Answer from the drawing. Dimensions are ordinates in mm from the lowest x, y and z of the part. A direction names the side the tool comes from. Coordinates: 2 decimals unless noted, no trailing zeros.
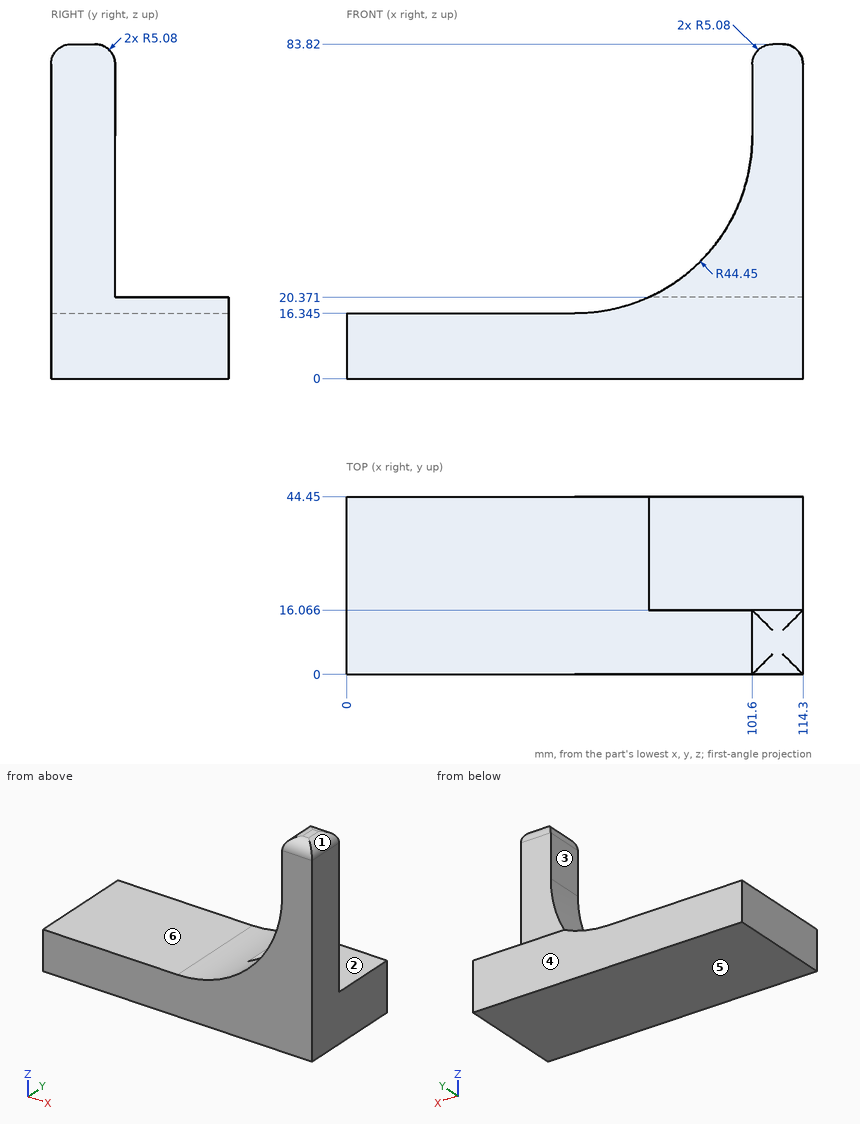
Item 1: Given pin 1 (17.5 mm diameter, centred on y = 8.5, z = 74, fed in from -X); pin 2 (19.5 mm diameter, centred on x = 96, z = 59.5, fed in from +Y) (1 decimal); pin 3 (8.5 mm diameter, centred on x = 92, y = 28, fed in from +Z), each flat-ended and moving along its own axis, determine where each tip first touches the part or whether it passes through.
Numbers:
pin 1: stops at x = 101.6
pin 2: stops at y = 16.1
pin 3: stops at z = 20.37
Item 2: Find the intervals of material crossed by line 1 along Z through (x, y) = (38.5, 19) (1 decimal); line 2 along Y through (x, z) = (103, 40) (1 decimal); line 3 along X through (y, z) = (4.5, 76), in increasing order.
Numbers:
line 1: z = 0 to 16.3
line 2: y = 0 to 16.1
line 3: x = 101.6 to 114.3
Item 3: Which of the six approach directions +Z, -Z, +X, -X, +Y, -Y give full straight-line access (tool end or side, diameter ignored) to the marked faces 1, 2 and 3?
Numbers:
face 1: +Z, +X, +Y, -Y
face 2: +Z, +X, -X, +Y
face 3: +Z, -X, +Y, -Y
Item 4: Determine the mould class of the marked faces 4, 5 and 6 for opening direction Z: released by +Z, released by -Z, zero draft, split by the parting line, or undercut.
Numbers:
face 4: zero draft
face 5: released by -Z
face 6: released by +Z
